Answer from the drawing. Dimensions are ordinates in mm from the lowest x, y and z of the part. A direction names the side the tool comes from. Give positions to 0.01 mm unless a question says otherwise; leave off trailing zeros. Order: outer loops, then holes, each group sorted by start corner. A loop starts at its lowest first (then second) coordinate and runs counter-clockwise, first axis right, second up. Notation, with made-up numbers: (50, -36) - (79, -36) arc R33 ccw to (79, 2) - close; hole circle Ø2 at (34.25, 40.5). An arc over 180 degrees is marked (long way). Use a Markdown table: item, result. Add a question column.
1) For the marked faces 1, 2 and 3, determine the directions among +Z, -Z, +X, -X, +Y, -Y from which every point of the face is accessible in a straight line to the end or side of a thin tool.
2) Find section D-D, the plane z = 12.5. Determine the outline of the cut face in (x, y).
3) Find section C-C, the plane z = 31. Determine the outline of the cut face in (x, y).
4) Flat-ended cylindrical pins translate along their axes: pin 1 (1 mm diameter, centred on y = 9, z = 77.5, fed in from -X) (1 decimal); pin 2 (1 mm diameter, centred on x = 85.5, z = 26, fed in from -Y); pin 3 (3 mm diameter, centred on x = 48, y = 22, fed in from +Z); pin 4 (8 mm diameter, centred on x = 30, y = 18.5, fed in from +Z). Find the tip coordinate at first contact, or state that the pin passes through.
5) Find section B-B, the plane y = 22. Determine the outline of the cut face in (x, z) (1 decimal).
6) Straight lines are drawn through the part: line 1 (X direction, y = 21.5, z = 32.5) (1 decimal); line 2 (X direction, y = 5, z = 85) (1 decimal); line 3 (Z direction, x = 56, y = 16.75) (1 decimal). For each, find the intervals that lie inside material, in ascending order.
7) The mould has two halves that part along X. Classify the marked faces 4, 5, 6 and 7: released by +X, released by -X, zero draft, split by the parting line, or undercut.
8) Find section A-A, the plane x = 50.8. Determine the outline of the cut face in (y, z) (1 decimal), plus the area to 3 significant figures.
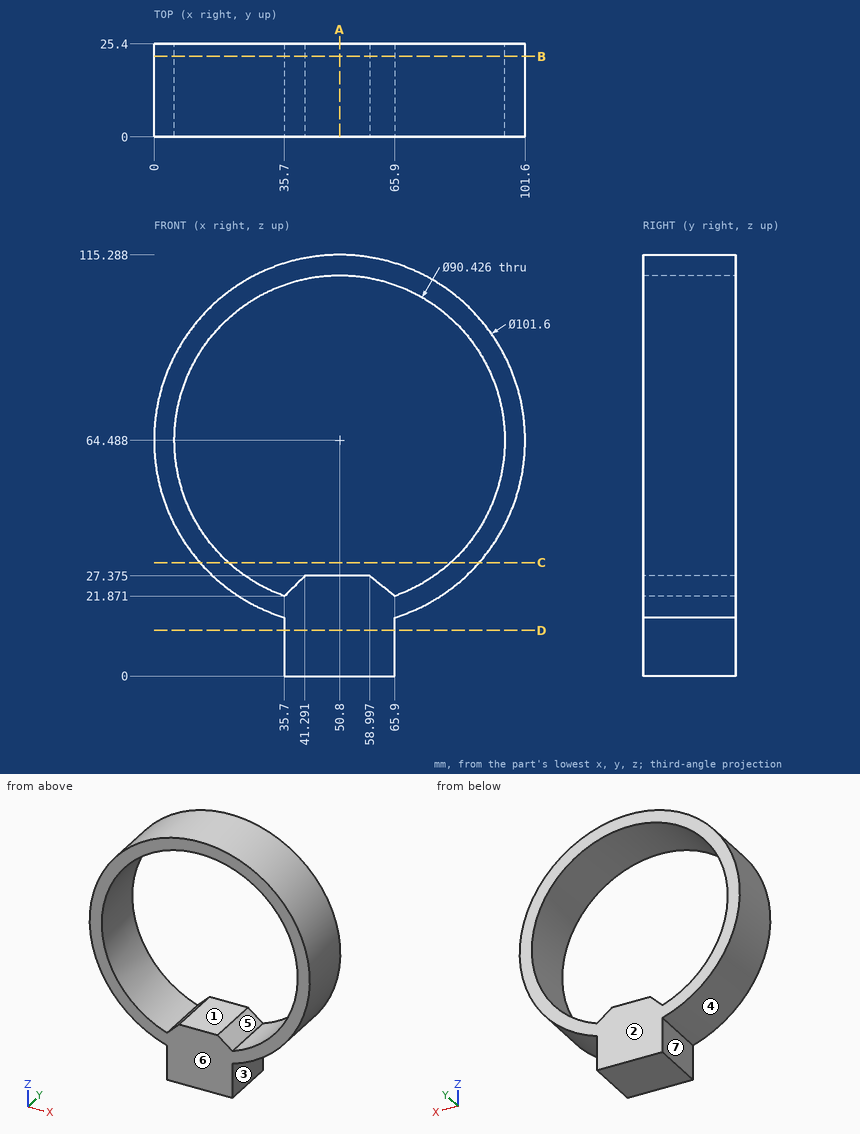
The answers:
| question | item | result |
|---|---|---|
| 1 | face 1 | +Y, -Y |
| 1 | face 2 | +Z, -Z, +X, -X, +Y |
| 1 | face 3 | -Z, +X, +Y, -Y |
| 2 | outline | (35.7, 0) - (65.9, 0) - (65.9, 25.4) - (35.7, 25.4) - close |
| 3 | outline | (12.6, 0) - (20.42, 0) - (20.42, 25.4) - (12.6, 25.4) - close; (81.18, 0) - (89, 0) - (89, 25.4) - (81.18, 25.4) - close |
| 4 | pin 1 | x = 1.6 |
| 4 | pin 2 | through |
| 4 | pin 3 | z = 115.27 |
| 4 | pin 4 | z = 112.43 |
| 5 | outline | (35.7, 0) - (65.9, 0) - (65.9, 16) arc R50.8 ccw (long way) to (35.7, 16) - close; hole (35.7, 21.9) - (41.3, 27.4) - (59, 27.4) - (65.9, 21.9) arc R45.2 ccw (long way) to start |
| 6 | line 1 | 11.3 to 18.8, 82.8 to 90.3 |
| 6 | line 2 | 4.3 to 10.5, 91.1 to 97.3 |
| 6 | line 3 | 0 to 27.4, 109.4 to 115 |
| 7 | face 4 | split by the parting line |
| 7 | face 5 | undercut |
| 7 | face 6 | zero draft |
| 7 | face 7 | released by -X |
| 8 | outline | (0, 0) - (25.4, 0) - (25.4, 27.4) - (0, 27.4) - close; (0, 109.7) - (25.4, 109.7) - (25.4, 115.3) - (0, 115.3) - close |
| 8 | area | 837 mm2 |
